from build123d import *

# Parameters (mm, degrees)
F0_R     = 2.3
F1_DEPTH = 8
F2_R     = 2.3
F3_DEPTH = 36.001
F4_R     = 1
F5_SIZE  = 0.5
F6_R     = 0.5


with BuildPart() as f1:
    # F0 (on Top) → F1 (new body)
    with BuildSketch(Plane.XY):
        with BuildLine():
            Line((18, 0), (0, 0))
            Line((0, 0), (-18, 0))
            Line((-18, 0), (-18, -20))
            Line((-18, -20), (-7.7, -20))
            Line((-7.7, -20), (-7.7, -11))
            ThreePointArc((-7.7, -11), (-7.4071067812, -10.2928932188), (-6.7, -10))
            Line((-6.7, -10), (0, -10))
            Line((0, -10), (6.7, -10))
            ThreePointArc((6.7, -10), (7.4071067812, -10.2928932188), (7.7, -11))
            Line((7.7, -11), (7.7, -20))
            Line((7.7, -20), (18, -20))
            Line((18, -20), (18, 0))
        make_face()
        with Locations((-13, -5)):
            Circle(F0_R, mode=Mode.SUBTRACT)
        with Locations((13, -5)):
            Circle(F0_R, mode=Mode.SUBTRACT)
    extrude(amount=F1_DEPTH)

    # F2 (on face) → F3 (cut, through all)
    with BuildSketch(Plane.YZ.offset(18)):
        with Locations((-16, 4)):
            Circle(F2_R)
    extrude(amount=-F3_DEPTH, mode=Mode.SUBTRACT)

    # F4
    f4_edges = [f1.edges().sort_by_distance(p)[0] for p in [
        (-18, -20, 4),
        (7.7, -20, 4),
        (18, -20, 4),
        (-18, 0, 4),
        (18, 0, 4),
        (-7.7, -20, 4),
    ]]
    fillet(f4_edges, radius=F4_R)

    # F5
    f5_edges = [f1.edges().sort_by_distance(p)[0] for p in [
        (-15.3, -5, 8),
        (10.7, -5, 8),
        (-15.3, -5, 0),
        (10.7, -5, 0),
        (-7.7, -18.3, 4),
        (-18, -18.3, 4),
        (7.7, -18.3, 4),
        (18, -18.3, 4),
    ]]
    chamfer(f5_edges, length=F5_SIZE)

    # F6
    f6_edges = [f1.edges().sort_by_distance(p)[0] for p in [
        (-12.85, -20, 8),
        (-7.992893, -19.707107, 8),
        (-7.7, -15, 8),
        (-7.407107, -10.292893, 8),
        (0, -10, 8),
        (7.407107, -10.292893, 8),
        (7.7, -15, 8),
        (7.992893, -19.707107, 8),
        (12.85, -20, 8),
        (17.707107, -19.707107, 8),
        (18, -10, 8),
        (17.707107, -0.292893, 8),
        (0, 0, 8),
        (-17.707107, -0.292893, 8),
        (-18, -10, 8),
        (-17.707107, -19.707107, 8),
        (-7.7, -15, 0),
    ]]
    fillet(f6_edges, radius=F6_R)


solid = f1.part
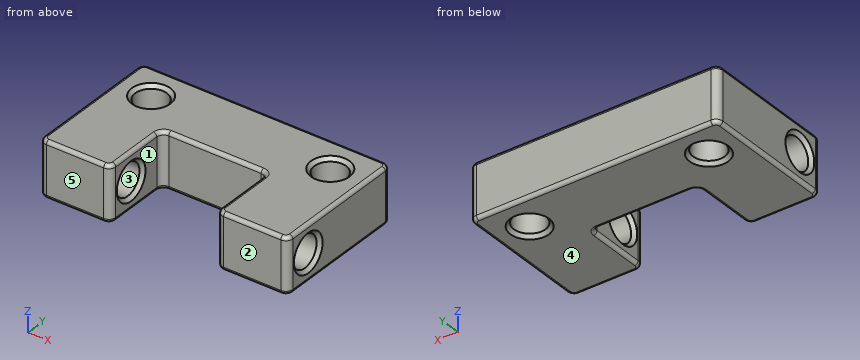
Geometry: final body of the model. Coordinates: model frame, mm. Face numbers are marked on the shaded views. A direction names the side the tool comes from. Coordinates: 2 decimals unless noted, no trailing zeros. Loops run counter-clockwise (first coordinate to the right, second up) from the corner with the lowest first, then second, coordinate; pieces in that order, holes last. Notation, with made-up numbers: M -12.5,-9 L 7.5,-9 A10 ccw 7.5,9 Z; hole C 48.5,16 d7. An arc over 180 degrees is marked long. One line per item, written item: value. Start each with the question number.
1) Pin query (flat end, axial travel): P1, Ø4, axis at y = -16, z = 4, coming from the -X side. Return the tip coordinate at first contact, or that it passes through.
2) Cut plane A-A (x = 13). Return loops of the section in (y, z).
3) Cut plane D-D (x = 0.5). Return loops of the section in (y, z).
4) Material intervals for L1, parallel to Z at x = -11, y = -16; L2, parallel to X at y = -6, z = 1.5; L3, parallel to Y at x = 13, z = 4.75, sorted ascending. Write a range as from..to.
5) Draft query along Z for the marked faces 3, 4 and 5. Return one class per face: released by +Z, released by -Z, zero draft, split by the parting line, or undercut.
6) Cut plane C-C (y = -12.5). Return loops of the section in (x, z), then the cut area to 3 significant figures.
7) Reachability of the marked faces 1 and 2 from +Z, -Z, +X, -X, +Y, -Y: full face, straight path, thin tool, end or side. Return the list, or none.
8) Cut plane B-B (y = -5). Return loops of the section in (x, z), then the cut area to 3 significant figures.
Evaluation:
1. P1: through
2. outline: M -20,0.5 A0.5 ccw -19.5,0 L -7.8,0 L -7.3,0.5 L -7.3,7.5 L -7.8,8 L -19.5,8 A0.5 ccw -20,7.5 Z; M -2.7,0.5 L -2.2,0 L -0.5,0 A0.5 ccw 0,0.5 L 0,7.5 A0.5 ccw -0.5,8 L -2.2,8 L -2.7,7.5 Z; hole C -16,4 d4.6
3. outline: M -10,0.5 A0.5 ccw -9.5,0 L -0.5,0 A0.5 ccw 0,0.5 L 0,7.5 A0.5 ccw -0.5,8 L -9.5,8 A0.5 ccw -10,7.5 Z
4. L1: 0..1.7, 6.3..8
4. L2: -18..-15.07, -10.93..10.93, 15.07..18
4. L3: -20..-18.17, -13.83..-7.3, -2.7..0
5. face 3: undercut
5. face 4: released by -Z
5. face 5: zero draft
6. outline: M -18,0.5 A0.5 ccw -17.5,0 L -8.2,0 A0.5 ccw -7.7,0.5 L -7.7,7.5 A0.5 ccw -8.2,8 L -17.5,8 A0.5 ccw -18,7.5 Z; M 7.7,0.5 A0.5 ccw 8.2,0 L 17.5,0 A0.5 ccw 18,0.5 L 18,7.5 A0.5 ccw 17.5,8 L 8.2,8 A0.5 ccw 7.7,7.5 Z
6. area: 164 mm^2
7. face 1: +Z, -Z, -Y
7. face 2: +Z, -Z, +X, -X, -Y
8. outline: M -18,0.5 A0.5 ccw -17.5,0 L -15.8,0 L -15.3,0.5 L -15.3,7.5 L -15.8,8 L -17.5,8 A0.5 ccw -18,7.5 Z; M -10.7,0.5 L -10.2,0 L 10.2,0 L 10.7,0.5 L 10.7,7.5 L 10.2,8 L -10.2,8 L -10.7,7.5 Z; M 15.3,0.5 L 15.8,0 L 17.5,0 A0.5 ccw 18,0.5 L 18,7.5 A0.5 ccw 17.5,8 L 15.8,8 L 15.3,7.5 Z
8. area: 213 mm^2
